Geometry: see drawing. Coordinates: mm, zero at the bounding-box minimum. A direction names the side the tool comes from. Give positions to 0.01 mm unless a question says otherwise; leave off trailing zeros. Write each loop counter-clockwise with the first axis right and the second up, starting at its lowest first coordinate (ties: lowest second). Pieces come first, ordered by that corner, then holes. Notation, with made-up numbers: (-34.5, -15) -> (-29.5, -15) arc R30 cw to (-29.5, 16) -> close; hole circle Ø4 at (62.25, 71.25). An arc over 180 degrees is marked (long way). Use one line per item in the form item = value. Start each with the question number.
(1) Cut plane B-B, the plane y = 14. Output: boundary loops of the cut face in (x, z), and give its area (3 significant figures).
(2) Set-up query: the marked faces 4 and 5. Return all of +Z, -Z, +X, -X, +Y, -Y with unobstructed straight access to the full face (end or side cutting, diameter ignored); none if empty.
(3) Cut plane A-A, the plane x = 14. Output: boundary loops of the cut face in (y, z).
(4) Material intervals for line 1 along Y through (x, z) = (15.25, 1.75) (1 decimal); line 2 along Z through (x, y) = (2.75, 19); line 3 along Y through (x, z) = (11.5, 2.5) (1 decimal), sorted ascending. Write a range as from..to.
(5) Cut plane C-C, the plane z = 4. Output: boundary loops of the cut face in (x, y).
(6) Draft query along X for the marked faces 1, 2 and 3. Return one class per face: pulls with the +X half, pulls with the -X half, needs draft (parallel to the pull), parting line crosses it, or undercut.
(7) Cut plane D-D, the plane y = 20. Output: boundary loops of the cut face in (x, z).
(8) First-contact query: P1, Ø3, axis at x = 17, z = 1.5, coming from the -Y side; P2, Ø1.5, axis at x = 15, z = 4.5, coming from the -Y side; P3, Ø4, axis at y = 11, z = 10.5, coming from the +X side; P4, Ø2.5, axis at x = 14, y = 14, coming from the -Z side. Flat tips, straight axial feed; report the tip coordinate or a pass-through.
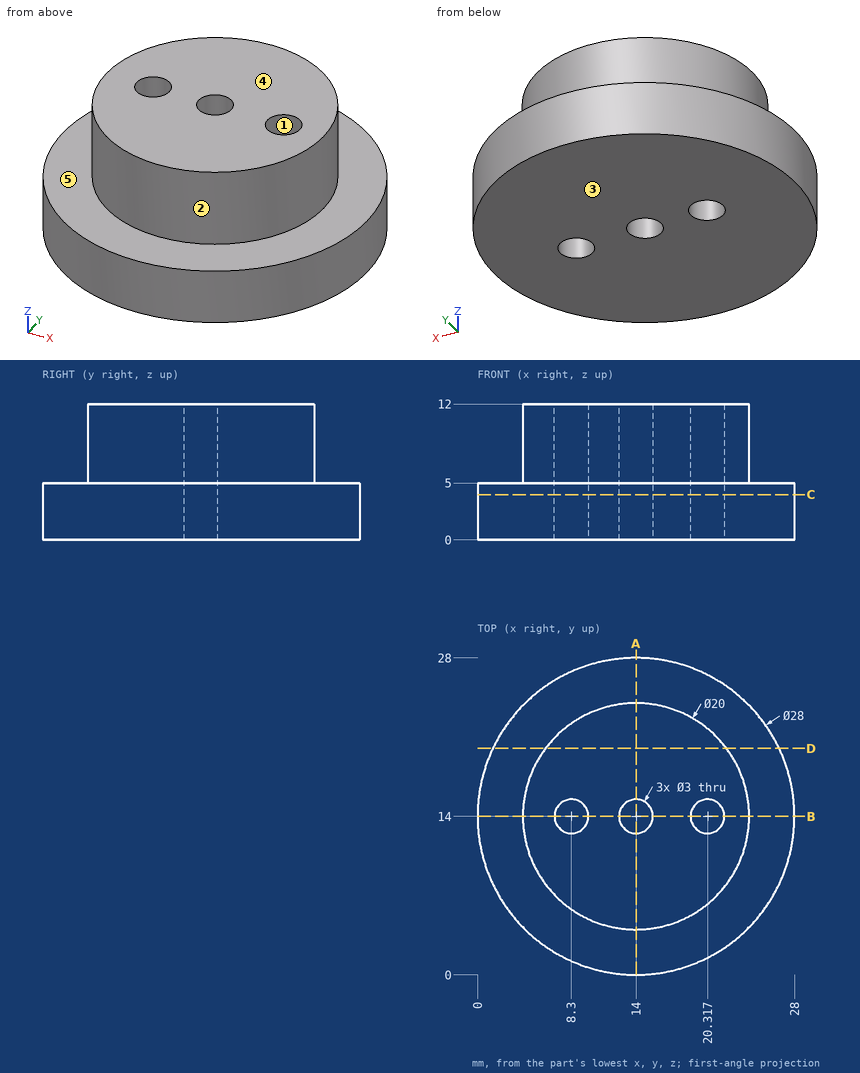
Geometry says:
q1.outline = (0, 0) -> (6.8, 0) -> (6.8, 12) -> (4, 12) -> (4, 5) -> (0, 5) -> close; (9.8, 0) -> (12.5, 0) -> (12.5, 12) -> (9.8, 12) -> close; (15.5, 0) -> (18.82, 0) -> (18.82, 12) -> (15.5, 12) -> close; (21.82, 0) -> (28, 0) -> (28, 5) -> (24, 5) -> (24, 12) -> (21.82, 12) -> close
q1.area = 172 mm^2
q2.face_4 = +Z, +X, -X, +Y, -Y
q2.face_5 = +Z
q3.outline = (0, 0) -> (12.5, 0) -> (12.5, 12) -> (4, 12) -> (4, 5) -> (0, 5) -> close; (15.5, 0) -> (28, 0) -> (28, 5) -> (24, 5) -> (24, 12) -> (15.5, 12) -> close
q4.line_1 = 0.1..13.2, 14.8..27.9
q4.line_2 = 0..5
q4.line_3 = 0.2..27.8
q5.outline = circle Ø28 at (14, 14); hole circle Ø3 at (8.3, 14); hole circle Ø3 at (14, 14); hole circle Ø3 at (20.32, 14)
q6.face_1 = undercut
q6.face_2 = parting line crosses it
q6.face_3 = needs draft
q7.outline = (1.35, 0) -> (26.65, 0) -> (26.65, 5) -> (22, 5) -> (22, 12) -> (6, 12) -> (6, 5) -> (1.35, 5) -> close
q8.P1 = 0.08
q8.P2 = 0
q8.P3 = 23.95
q8.P4 = through
